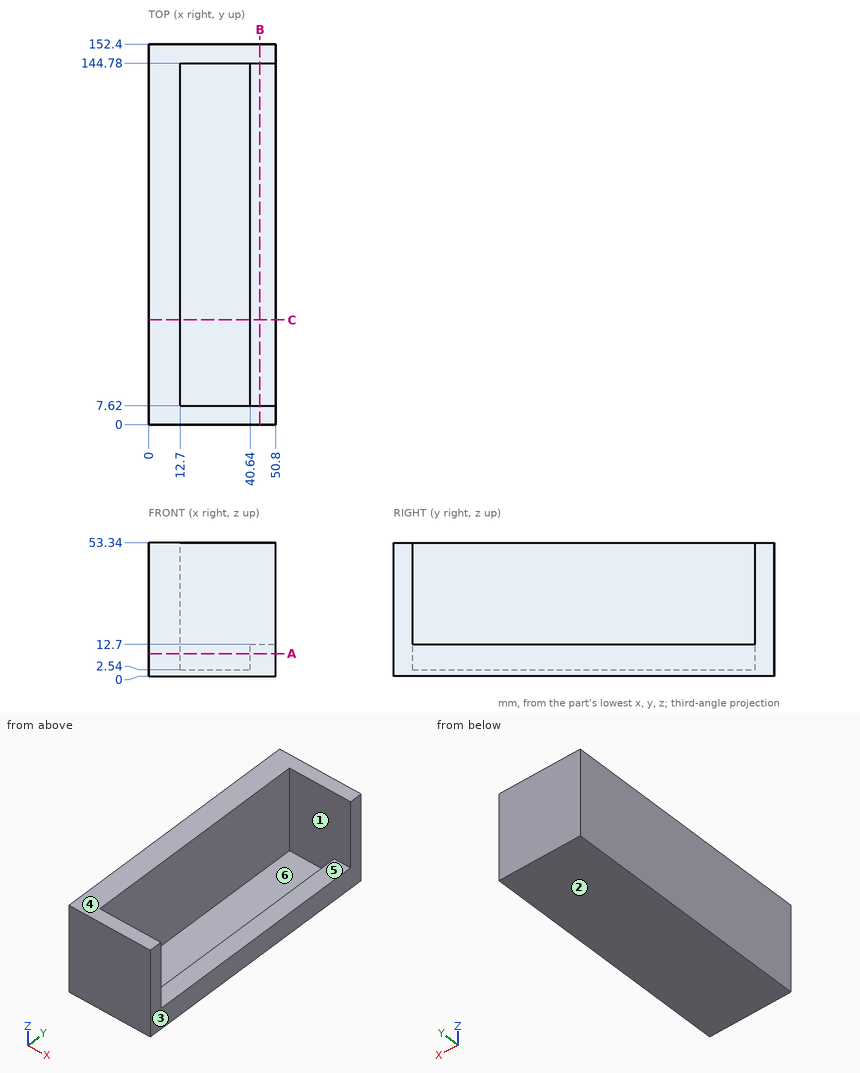
Check sheet for the drawn part. Datum: minimum x, y, z corner. Units: mm. A direction names the side the tool comes from. Give positions to 0.01 mm unless a question says otherwise; leave off trailing zeros. Loops run counter-clockwise (first coordinate to the right, second up) from the corner with the lowest first, then second, coordinate; pieces in that order, holes last.
1) Sectioned sample at B-B, the plane x = 44.5. Enter the section's corners in (y, z).
2) Draft check along X on the marked faces 1, 2 and 3. Enter one of: pulls with the +X half, pulls with the -X half, needs draft (parallel to the pull), parting line crosses it, or undercut.
3) Depth check by flat-ended pin: pin 1 Ø1 at (y, z) = (98, 18.5) entering from +X; pin 2 Ø5 at (x, y) = (47, 87) entering from +Z. Enter the tip coordinate at first touch or a pass-through.
4) Sectioned sample at A-A, the plane z = 9. Enter the section's corners in (x, y), then the cut area to 3 significant figures.
5) Sectioned sample at C-C, the plane y = 42. Enter the section's corners in (x, z).
6) Thickness scan on line 1 along X through (y, z) = (97, 5); line 2 along Y through (x, z) = (31, 10.5); line 3 along X through (y, z) = (48.5, 43). Record the ranges inside material, lowest first.
7) Set-up check for the marked faces 4, 5 and 6: record each of +Z, -Z, +X, -X, +Y, -Y from which the full face is reachable in a straight line by a thin tool's end or side.
Answers:
1. outline: (0, 0) - (152.4, 0) - (152.4, 53.34) - (144.78, 53.34) - (144.78, 12.7) - (7.62, 12.7) - (7.62, 53.34) - (0, 53.34) - close
2. face 1: undercut
2. face 2: needs draft
2. face 3: pulls with the +X half
3. pin 1: stops at x = 12.7
3. pin 2: stops at z = 12.7
4. outline: (0, 0) - (50.8, 0) - (50.8, 152.4) - (0, 152.4) - close; hole (12.7, 7.62) - (40.64, 7.62) - (40.64, 144.78) - (12.7, 144.78) - close
4. area: 3,910 mm2
5. outline: (0, 0) - (50.8, 0) - (50.8, 12.7) - (40.64, 12.7) - (40.64, 2.54) - (12.7, 2.54) - (12.7, 53.34) - (0, 53.34) - close
6. line 1: x = 0 to 12.7, 40.64 to 50.8
6. line 2: y = 0 to 7.62, 144.78 to 152.4
6. line 3: x = 0 to 12.7
7. face 4: +Z, +X, -X, +Y, -Y
7. face 5: +Z, +X
7. face 6: +Z
